```python
from build123d import *

# Parameters (mm, degrees)
SKETCH_1_W                  = 350
SKETCH_1_H                  = 260
EXTRUDE_1_DEPTH             = 3
FILLET_2_R                  = 30
CUT_EXTRUDE_2_REACH         = 220.023
SKETCH_3_R                  = 22
PATTERN_LINEAR_1_COUNT      = 2
PATTERN_LINEAR_1_PITCH      = 85
PATTERN_LINEAR_1_COUNT_DIR2 = 3
PATTERN_LINEAR_1_PITCH_DIR2 = 85
MIRROR_1_COPY_1_REACH       = 220.023
MIRROR_1_COPY_1_SKETCH_R    = 22
MIRROR_1_COPY_2_REACH       = 220.023
MIRROR_1_COPY_2_SKETCH_R    = 22
MIRROR_1_COPY_3_REACH       = 220.023
MIRROR_1_COPY_3_SKETCH_R    = 22
MIRROR_1_COPY_4_REACH       = 220.023
MIRROR_1_COPY_4_SKETCH_R    = 22
MIRROR_1_COPY_5_REACH       = 220.023
MIRROR_1_COPY_5_SKETCH_R    = 22
CUT_EXTRUDE_3_REACH         = 220.023
SKETCH_4_W                  = 48.4
SKETCH_4_H                  = 24.5
FILLET_3_R                  = 2


with BuildPart() as part:
    # 草圖1 → 填料-伸長1 (new body)
    with BuildSketch(Plane(origin=(0, 0, 0), x_dir=(1, 0, 0), z_dir=(0, 1, 0))):
        Rectangle(SKETCH_1_W, SKETCH_1_H)
    extrude(amount=EXTRUDE_1_DEPTH)

    # 圓角2
    fillet_2_edges = [part.edges().sort_by_distance(p)[0] for p in [
        (175, 1.5, 130),
        (-175, 1.5, 130),
        (-175, 1.5, -130),
        (175, 1.5, -130),
    ]]
    fillet(fillet_2_edges, radius=FILLET_2_R)

    # 草圖3 → 除料-伸長2 (cut, up to next)
    with BuildSketch(Plane(origin=(0, 3, 0), x_dir=(1, 0, 0), z_dir=(0, 1, 0)), mode=Mode.PRIVATE) as cut_extrude_2_sk1:
        with Locations(Location((-132.5, 85, 0), (0, 0, 270))):
            Circle(SKETCH_3_R)
    cut_extrude_2_tool1 = extrude(cut_extrude_2_sk1.sketch, amount=-CUT_EXTRUDE_2_REACH, mode=Mode.PRIVATE) & part.part
    cut_extrude_2 = cut_extrude_2_tool1.solids().sort_by_distance((-132.5, 3, -85))[0]
    add(cut_extrude_2, mode=Mode.SUBTRACT)

    # 直線複製排列1: Cut-Extrude 2 2 × 3
    with Locations(*[(i * PATTERN_LINEAR_1_PITCH, 0, j * PATTERN_LINEAR_1_PITCH_DIR2) for i in range(PATTERN_LINEAR_1_COUNT) for j in range(PATTERN_LINEAR_1_COUNT_DIR2) if (i, j) != (0, 0)]):
        add(cut_extrude_2, mode=Mode.SUBTRACT)

    # 鏡射1: 除料-伸長2 across plane
    add(cut_extrude_2.mirror(Plane(origin=(0, 0, 0), x_dir=(0, 0, 1), z_dir=(1, 0, 0))), mode=Mode.SUBTRACT)

    # 鏡射1 copy 1 sketch → 鏡射1 copy 1 (cut, up to next)
    with BuildSketch(Plane(origin=(0, 3, 85), x_dir=(-1, 0, 0), z_dir=(0, 1, 0)), mode=Mode.PRIVATE) as mirror_1_copy_1_sk1:
        with Locations((-132.5, -85)):
            Circle(MIRROR_1_COPY_1_SKETCH_R)
    mirror_1_copy_1_tool1 = extrude(mirror_1_copy_1_sk1.sketch, amount=-MIRROR_1_COPY_1_REACH, mode=Mode.PRIVATE) & part.part
    add(mirror_1_copy_1_tool1.solids().sort_by_distance((132.5, 3, 0))[0], mode=Mode.SUBTRACT)

    # 鏡射1 copy 2 sketch → 鏡射1 copy 2 (cut, up to next)
    with BuildSketch(Plane(origin=(0, 3, 170), x_dir=(-1, 0, 0), z_dir=(0, 1, 0)), mode=Mode.PRIVATE) as mirror_1_copy_2_sk1:
        with Locations((-132.5, -85)):
            Circle(MIRROR_1_COPY_2_SKETCH_R)
    mirror_1_copy_2_tool1 = extrude(mirror_1_copy_2_sk1.sketch, amount=-MIRROR_1_COPY_2_REACH, mode=Mode.PRIVATE) & part.part
    add(mirror_1_copy_2_tool1.solids().sort_by_distance((132.5, 3, 85))[0], mode=Mode.SUBTRACT)

    # 鏡射1 copy 3 sketch → 鏡射1 copy 3 (cut, up to next)
    with BuildSketch(Plane(origin=(-85, 3, 0), x_dir=(-1, 0, 0), z_dir=(0, 1, 0)), mode=Mode.PRIVATE) as mirror_1_copy_3_sk1:
        with Locations((-132.5, -85)):
            Circle(MIRROR_1_COPY_3_SKETCH_R)
    mirror_1_copy_3_tool1 = extrude(mirror_1_copy_3_sk1.sketch, amount=-MIRROR_1_COPY_3_REACH, mode=Mode.PRIVATE) & part.part
    add(mirror_1_copy_3_tool1.solids().sort_by_distance((47.5, 3, -85))[0], mode=Mode.SUBTRACT)

    # 鏡射1 copy 4 sketch → 鏡射1 copy 4 (cut, up to next)
    with BuildSketch(Plane(origin=(-85, 3, 85), x_dir=(-1, 0, 0), z_dir=(0, 1, 0)), mode=Mode.PRIVATE) as mirror_1_copy_4_sk1:
        with Locations((-132.5, -85)):
            Circle(MIRROR_1_COPY_4_SKETCH_R)
    mirror_1_copy_4_tool1 = extrude(mirror_1_copy_4_sk1.sketch, amount=-MIRROR_1_COPY_4_REACH, mode=Mode.PRIVATE) & part.part
    add(mirror_1_copy_4_tool1.solids().sort_by_distance((47.5, 3, 0))[0], mode=Mode.SUBTRACT)

    # 鏡射1 copy 5 sketch → 鏡射1 copy 5 (cut, up to next)
    with BuildSketch(Plane(origin=(-85, 3, 170), x_dir=(-1, 0, 0), z_dir=(0, 1, 0)), mode=Mode.PRIVATE) as mirror_1_copy_5_sk1:
        with Locations((-132.5, -85)):
            Circle(MIRROR_1_COPY_5_SKETCH_R)
    mirror_1_copy_5_tool1 = extrude(mirror_1_copy_5_sk1.sketch, amount=-MIRROR_1_COPY_5_REACH, mode=Mode.PRIVATE) & part.part
    add(mirror_1_copy_5_tool1.solids().sort_by_distance((47.5, 3, 85))[0], mode=Mode.SUBTRACT)

    # 草圖4 → 除料-伸長3 (cut, up to next)
    with BuildSketch(Plane(origin=(0, 3, 0), x_dir=(1, 0, 0), z_dir=(0, 1, 0)), mode=Mode.PRIVATE) as cut_extrude_3_sk1:
        with Locations((0, 117.75)):
            Rectangle(SKETCH_4_W, SKETCH_4_H)
    cut_extrude_3_tool1 = extrude(cut_extrude_3_sk1.sketch, amount=-CUT_EXTRUDE_3_REACH, mode=Mode.PRIVATE) & part.part
    add(cut_extrude_3_tool1.solids().sort_by_distance((0, 3, -117.75))[0], mode=Mode.SUBTRACT)

    # 圓角3
    fillet_3_edges = [part.edges().sort_by_distance(p)[0] for p in [
        (-24.2, 1.5, -105.5),
        (24.2, 1.5, -105.5),
    ]]
    fillet(fillet_3_edges, radius=FILLET_3_R)


solid = part.part
```
Work out the finished part from the listing and answer in its coordinate system (mm). Coordinates: 2 decimals unless noted, no trailing zeros. Loops run counter-clockwise (first coordinate to the right, second up) from the corner with the lowest first, then second, coordinate; pieces in that order, holes last. Notation, with made-up numbers: (71, 11.5) - (93, 11.5) arc R5 cw to (93, 18.5) - close; hole circle Ø6 at (48, 22.5). An arc over 180 degrees is marked (long way). Use a Markdown table: item, result.
Item 1: The mould has two halves that part along X. Classify faces 1 (the cylindrical face through (166.445, 1.521, -120.979)), 2 (the cylindrical face through (27.18, 1.52, -8.43)), 3 (the cylindrical face through (154.48, 1.52, 85.97)), 4 (the cylindrical face through (-166.445, 1.521, -120.979)): +X half, -X half, draft (parallel to the pull), parting line (faces both ways), or undercut.
Evaluation:
| item | result |
|---|---|
| face 1 | +X half |
| face 2 | undercut |
| face 3 | undercut |
| face 4 | -X half |
Item 2: Find section A-A, the plane z = 85. Determine the outline of the cut face in (x, y), and give its area (3 significant figures).
Evaluation:
| item | result |
|---|---|
| outline | (-175, 0) - (-154.5, 0) - (-154.5, 3) - (-175, 3) - close; (-110.5, 0) - (-69.5, 0) - (-69.5, 3) - (-110.5, 3) - close; (-25.5, 0) - (25.5, 0) - (25.5, 3) - (-25.5, 3) - close; (69.5, 0) - (110.5, 0) - (110.5, 3) - (69.5, 3) - close; (154.5, 0) - (175, 0) - (175, 3) - (154.5, 3) - close |
| area | 522 mm2 |
Item 3: Consider probe 1 along Z at (x, y) = (-54, 1.65); probe 2 along Z at (x, y) = (-137, 1.25); probe 3 along X at (y, z) = (2, 89). Determine where each line is inside the solid, lowest interval first. Write a range as from..to.
Evaluation:
| item | result |
|---|---|
| probe 1 | z = -130..-106.02, -63.98..-21.02, 21.02..63.98, 106.02..130 |
| probe 2 | z = -130..-106.53, -63.47..-21.53, 21.53..63.47, 106.53..130 |
| probe 3 | x = -175..-154.13, -110.87..-69.13, -25.87..25.87, 69.13..110.87, 154.13..175 |
Item 4: Find section B-B, the plane y = 1.7. State how many separate pieces and enclosed holes the cut face has, and give its area (3 significant figures).
Evaluation:
| item | result |
|---|---|
| separate pieces | 1 |
| enclosed holes | 12 |
| area | 70,800 mm2 |
Item 5: Given pin 1 Ø0.9 at (x, y) = (3, 1) entering from -Z; pin 2 Ø0.9 at (y, z) = (2, -121.5) entering from +X; pin 3 Ø0.9 at (y, z) = (1, -116.5) entering from -X, each flat-ended and moving along its own axis, determine where each tip first touches the part or whether it passes through.
Evaluation:
| item | result |
|---|---|
| pin 1 | stops at z = -105.5 |
| pin 2 | stops at x = 166.38 |
| pin 3 | stops at x = -170.35 |
Item 6: Find section D-D, the plane x = 121. Determine the outline of the cut face in (y, z) (3 decimals), and give its area (3 significant figures).
Evaluation:
| item | result |
|---|---|
| outline | (0, -130) - (3, -130) - (3, -103.755) - (0, -103.755) - close; (0, -66.245) - (3, -66.245) - (3, -18.755) - (0, -18.755) - close; (0, 18.755) - (3, 18.755) - (3, 66.245) - (0, 66.245) - close; (0, 103.755) - (3, 103.755) - (3, 130) - (0, 130) - close |
| area | 442 mm2 |
Item 7: Find section C-C, the plane x = -47.5. Determine the outline of the cut face in (y, z), and give its area (3 significant figures).
Evaluation:
| item | result |
|---|---|
| outline | (0, -130) - (3, -130) - (3, -107) - (0, -107) - close; (0, -63) - (3, -63) - (3, -22) - (0, -22) - close; (0, 22) - (3, 22) - (3, 63) - (0, 63) - close; (0, 107) - (3, 107) - (3, 130) - (0, 130) - close |
| area | 384 mm2 |
